```python
from build123d import *

# Parameters (mm, degrees)
BOSS_EXTRUDE1_DEPTH = 3.8
SKETCH2_2_R         = 1.75
CUT_EXTRUDE1_DEPTH  = 1.9
SKETCH3_R           = 0.375
BOSS_EXTRUDE3_DEPTH = 7.75


with BuildPart() as part:
    # Sketch1 → Boss-Extrude1 (new body)
    with BuildSketch(Plane(origin=(0, 0, 0), x_dir=(1, 0, 0), z_dir=(0, 1, 0))):
        with BuildLine():
            Line((0.75, 0), (9.75, 0))
            ThreePointArc((9.75, 0), (10.280330086, 0.219669914), (10.5, 0.75))
            Line((10.5, 0.75), (10.5, 9.75))
            ThreePointArc((10.5, 9.75), (10.280330086, 10.280330086), (9.75, 10.5))
            Line((9.75, 10.5), (0.75, 10.5))
            ThreePointArc((0.75, 10.5), (0.219669914, 10.280330086), (0, 9.75))
            Line((0, 9.75), (0, 0.75))
            ThreePointArc((0, 0.75), (0.219669914, 0.219669914), (0.75, 0))
        make_face()
    extrude(amount=BOSS_EXTRUDE1_DEPTH)

    # Sketch2_2 → Cut-Extrude1 (cut)
    with BuildSketch(Plane(origin=(0, 3.8, 0), x_dir=(1, 0, 0), z_dir=(0, 1, 0))):
        with Locations(Location((5.25, 5.25, 0), (0, 0, 270))):
            Circle(SKETCH2_2_R)
    extrude(amount=-CUT_EXTRUDE1_DEPTH, mode=Mode.SUBTRACT)

    # Sketch3 → Boss-Extrude3 (add)
    with BuildSketch(Plane.XZ):
        with Locations(Location((9.45, -1.05, 0), (0, 0, 270))):
            Circle(SKETCH3_R)
        with Locations(Location((9.45, -9.45, 0), (0, 0, 270))):
            Circle(SKETCH3_R)
        with Locations(Location((1.05, -9.45, 0), (0, 0, 270))):
            Circle(SKETCH3_R)
        with Locations(Location((1.05, -1.05, 0), (0, 0, 270))):
            Circle(SKETCH3_R)
    extrude(amount=BOSS_EXTRUDE3_DEPTH)


solid = part.part
```
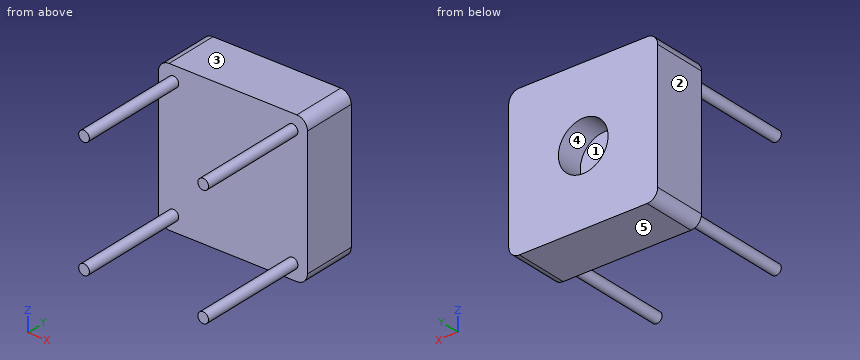
Read the model definition and answer for the solid it produces. Units are mm, in the model's axes. Face numbers are marked on the shaded views. A direction names the side the tool comes from. Coordinates: 2 decimals unless noted, no trailing zeros. Order: outer loops, then holes, each group sorted by start corner. A loop starts at its lowest first (then second) coordinate and runs counter-clockwise, first axis right, second up. Notation, with made-up numbers: (86.5, -30.75) - (137.5, -30.75) arc R20 ccw to (137.5, -6.75) - close; hole circle Ø3 at (89.5, -1). An arc over 180 degrees is marked (long way). Answer as a JSON object with one key per item and string values. Group by question number.
Item 1: Section B-B (x = 5.25) is taken. Give the vertices of the cut face in (y, z).
Item 2: Section D-D (z = -5.25) is taken. Give the vertices of the cut face in (x, y).
Item 3: Flat-ended cylindrical pins translate along their axes: P1, Ø1, axis at y = -1, z = -8.5, coming from the +X side; P2, Ø2, axis at x = 6.5, z = -9, coming from the -Y side; P3, Ø3, axis at x = 5.25, z = -5.25, coming from the +Y side. Find the tip coordinate at first contact, or state that the pin passes through.
Item 4: Section A-A (z = -9.45) is taken. Give the vertices of the cut face in (x, y) (3 decimals), plus the area to 3 significant figures.
Item 5: Section C-C (y = -5.75) is taken. Give the vertices of the cut face in (x, z) (3 decimals).
Item 6: Consider probe 1 along X at (y, z) = (3.15, -5.25); probe 2 along Y at (x, z) = (2.75, -3.5); probe 3 along Y at (x, z) = (6.5, -4.25). Determine where each line is inside the solid, lowest interval first. Write a range as from..to.
Item 7: A tool of negligible diameter and unlimited length cuts with its end or side. For the marked faces 1 and 2, from which of +Z, -Z, +X, -X, +Y, -Y can it reach the whole face along a straight path? Write none if from no direction.
Item 8: The mould has two halves that part along Z. Classify the marked faces 3, 4 and 5: +Z half, -Z half, draft (parallel to the pull), parting line (faces both ways), or undercut.
Results are:
{
 "1": {"outline": "(0, -10.5) - (3.8, -10.5) - (3.8, -7) - (1.9, -7) - (1.9, -3.5) - (3.8, -3.5) - (3.8, 0) - (0, 0) - close"},
 "2": {"outline": "(0, 0) - (10.5, 0) - (10.5, 3.8) - (7, 3.8) - (7, 1.9) - (3.5, 1.9) - (3.5, 3.8) - (0, 3.8) - close"},
 "3": {"P1": "passes through", "P2": "stops at y = 0", "P3": "stops at y = 1.9"},
 "4": {"outline": "(0, 0) - (0.675, 0) - (0.675, -7.75) - (1.425, -7.75) - (1.425, 0) - (9.075, 0) - (9.075, -7.75) - (9.825, -7.75) - (9.825, 0) - (10.5, 0) - (10.5, 3.8) - (0, 3.8) - close", "area": "51.5 mm^2"},
 "5": {"outline": "circle Ø0.75 at (1.05, -9.45); circle Ø0.75 at (1.05, -1.05); circle Ø0.75 at (9.45, -9.45); circle Ø0.75 at (9.45, -1.05)"},
 "6": {"probe 1": "x = 0..3.5, 7..10.5", "probe 2": "y = 0..3.8", "probe 3": "y = 0..1.9"},
 "7": {"face 1": "+Y", "face 2": "+Z, -Z, -X, +Y, -Y"},
 "8": {"face 3": "+Z half", "face 4": "undercut", "face 5": "-Z half"}
}
